```python
from build123d import *

# Parameters (mm, degrees)
SKETCH1_R           = 12.7
BOSS_EXTRUDE1_DEPTH = 12.7
SKETCH2_R           = 1.6256
CUT_EXTRUDE1_DEPTH  = 9.525
SKETCH3_R           = 9.525
CUT_EXTRUDE2_DEPTH  = 2.54
BOSS_EXTRUDE6_START = -12.7
BOSS_EXTRUDE6_DEPTH = 12.7
SKETCH15_R          = 12.7
BOSS_EXTRUDE8_DEPTH = 12.7
SKETCH17_R          = 1.651
CUT_EXTRUDE4_DEPTH  = 12.7
SKETCH18_R          = 3.81
CUT_EXTRUDE5_DEPTH  = 10.9027722
SKETCH19_R          = 8.255
CUT_EXTRUDE6_DEPTH  = 8.3627722
SKETCH20_R          = 9.525
CUT_EXTRUDE7_DEPTH  = 5.1877722
SKETCH21_R          = 1.2192
CUT_EXTRUDE8_DEPTH  = 4.3372278


with BuildPart() as part:
    # Sketch1 → Boss-Extrude1 (new body)
    with BuildSketch(Plane(origin=(0, 0, 0), x_dir=(1, 0, 0), z_dir=(0, 1, 0))):
        with Locations(Location((0, 0, 0), (0, 0, 270))):
            Circle(SKETCH1_R)
    extrude(amount=BOSS_EXTRUDE1_DEPTH)

    # Sketch2 → Cut-Extrude1 (cut)
    with BuildSketch(Plane.XZ):
        with Locations(Location((0, 0, 0), (0, 0, 270))):
            Circle(SKETCH2_R)
    extrude(amount=-CUT_EXTRUDE1_DEPTH, mode=Mode.SUBTRACT)

    # Sketch3 → Cut-Extrude2 (cut)
    with BuildSketch(Plane.XZ):
        with Locations(Location((0, 0, 0), (0, 0, 270))):
            Circle(SKETCH3_R)
    extrude(amount=-CUT_EXTRUDE2_DEPTH, mode=Mode.SUBTRACT)

    # Sketch14 → Boss-Extrude6 (add)
    with BuildSketch(Plane(origin=(0, 12.7, 0), x_dir=(1, 0, 0), z_dir=(0, 1, 0)).offset(BOSS_EXTRUDE6_START)):
        with BuildLine():
            Line((15.875, 12.7), (0, 12.7))
            ThreePointArc((0, 12.7), (8.980256121, 8.980256121), (12.7, 0))
            ThreePointArc((12.7, 0), (8.980256121, -8.980256121), (0, -12.7))
            Line((0, -12.7), (15.875, -12.7))
            Line((15.875, -12.7), (15.875, 12.7))
        make_face()
    extrude(amount=BOSS_EXTRUDE6_DEPTH)

    # Sketch5 → #2-56 Tapped Hole1 (revolve, cut)
    with BuildSketch(Plane(origin=(0, 3.81, 0), x_dir=(0, 1, 0), z_dir=(1, 0, 0))):
        Polygon((0, 0), (0, 13.74216509), (0.889, 13.208), (0.889, 0), align=None)
    revolve(axis=Axis((0, 3.81, -6.35), (0, 0, 1)), mode=Mode.SUBTRACT)

    # Sketch15 → Boss-Extrude8 (add)
    with BuildSketch(Plane(origin=(15.875, 0, 0), x_dir=(0, 0, -1), z_dir=(1, 0, 0))):
        with Locations((0, 25.4)):
            Circle(SKETCH15_R)
        with BuildLine():
            ThreePointArc((0, 12.7), (-8.980256121, 16.419743879), (-12.7, 25.4))
            Line((-12.7, 25.4), (-12.7, 12.7))
            Line((-12.7, 12.7), (0, 12.7))
        make_face()
        with BuildLine():
            Line((12.7, 12.7), (12.7, 25.4))
            ThreePointArc((12.7, 25.4), (8.980256121, 16.419743879), (0, 12.7))
            Line((0, 12.7), (12.7, 12.7))
        make_face()
    extrude(amount=-BOSS_EXTRUDE8_DEPTH)

    # Sketch17 → Cut-Extrude4 (cut)
    with BuildSketch(Plane.ZY.offset(-3.175)):
        with Locations((0, 25.4)):
            Circle(SKETCH17_R)
    extrude(amount=-CUT_EXTRUDE4_DEPTH, mode=Mode.SUBTRACT)

    # Sketch18 → Cut-Extrude5 (cut)
    with BuildSketch(Plane.ZY.offset(-3.175)):
        with Locations((0, 25.4)):
            Circle(SKETCH18_R)
    extrude(amount=-CUT_EXTRUDE5_DEPTH, mode=Mode.SUBTRACT)

    # Sketch19 → Cut-Extrude6 (cut)
    with BuildSketch(Plane.ZY.offset(-3.175)):
        with Locations((0, 25.4)):
            Circle(SKETCH19_R)
    extrude(amount=-CUT_EXTRUDE6_DEPTH, mode=Mode.SUBTRACT)

    # Sketch20 → Cut-Extrude7 (cut)
    with BuildSketch(Plane.ZY.offset(-3.175)):
        with Locations((0, 25.4)):
            Circle(SKETCH20_R)
    extrude(amount=-CUT_EXTRUDE7_DEPTH, mode=Mode.SUBTRACT)

    # Sketch21 → Cut-Extrude8 (cut)
    with BuildSketch(Plane.ZY.offset(-11.5377722)):
        with Locations((5.4599967, 25.4)):
            Circle(SKETCH21_R)
        with Locations((-5.4599967, 25.4)):
            Circle(SKETCH21_R)
    extrude(amount=-CUT_EXTRUDE8_DEPTH, mode=Mode.SUBTRACT)


solid = part.part
```
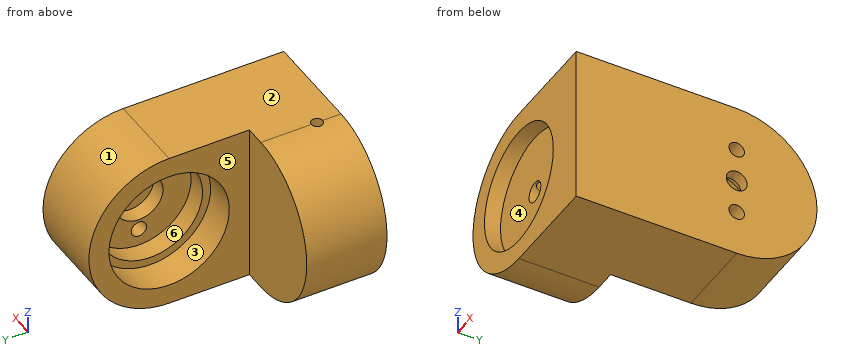
Design review of the part built by this model. Coordinates are the model's own, in mm. Face numbers are marked on the shaded views. A direction names the side the tool comes from. Round coordinates to 2 decimals unless told otherwise and drop trailing zeros. Write each loop counter-clockwise with the first axis right and the second up, starting at its lowest first coordinate (ties: lowest second). Pieces come first, ordered by that corner, then holes. Notation, with made-up numbers: (0, 77) -> (4, 77) arc R13 ccw to (4, 85) -> close; hole circle Ø6 at (75.5, 11.25). An arc over 180 degrees is marked (long way). Answer in a Markdown table with one row per item.
Q1. Draft analysis for pull direction Y (two halves, no side actions). For the marked faces 1, 2 and 3, state which applies: +Y half, -Y half, draft (parallel to the pull), parting line (faces both ways), or undercut.
The answers:
| item | result |
|---|---|
| face 1 | +Y half |
| face 2 | draft |
| face 3 | undercut |
Q2. For the marked faces 4, 5 and 6, list the 3-axis set-ups (+Z, -Z, +X, -X, +Y, -Y) from which the entire face can be reached by the end or side of a thin tool; tool diameter is ignored.
The answers:
| item | result |
|---|---|
| face 4 | -Y |
| face 5 | +Z, -Z, -X, +Y |
| face 6 | -X |
Q3. To check wall thickness, follow L1, parallel to Y at x = 15.3, z = 0; L2, parallel to Y at x = 12.3, z = 0; L3, parallel to X at y = 21, z = 2.75 (3 decimals). State the ranges of each line that lie inside material, in increasing order. Write a range as [from, to].
The answers:
| item | result |
|---|---|
| L1 | [0, 23.75], [27.05, 38.1] |
| L2 | [0, 21.59], [29.21, 38.1] |
| L3 | [11.538, 15.875] |
Q4. Take a section at B-B, the plane x = 12.75. State the section outline as (y, z) points.
The answers:
| item | result |
|---|---|
| outline | (0, -12.7) -> (25.4, -12.7) arc R12.7 ccw to (25.4, 12.7) -> (0, 12.7) -> close; hole circle Ø7.62 at (25.4, 0); hole circle Ø2.44 at (25.4, -5.46); hole circle Ø2.44 at (25.4, 5.46) |
Q5. Clearance check with flat-ended pins moving along their axes: pin 1 Ø12.5 at (y, z) = (22.5, 4) entering from -X (3 decimals); pin 2 Ø6 at (y, z) = (25.4, 0) entering from -X; pin 3 Ø4 at (x, z) = (0, 0) entering from +Y. State where each tip first meets the part, or that it passes through.
The answers:
| item | result |
|---|---|
| pin 1 | x = 3.175 |
| pin 2 | x = 14.08 |
| pin 3 | y = 12.7 |
Q6. Take a section at D-D, the plane y = 23. State the section outline as (x, z) points (3 decimals), then the cut area to 3 significant figures.
The answers:
| item | result |
|---|---|
| outline | (3.175, -12.7) -> (15.875, -12.7) -> (15.875, 12.7) -> (3.175, 12.7) -> (3.175, 9.218) -> (8.363, 9.218) -> (8.363, 7.898) -> (11.538, 7.898) -> (11.538, 2.959) -> (14.078, 2.959) -> (14.078, -2.959) -> (11.538, -2.959) -> (11.538, -7.898) -> (8.363, -7.898) -> (8.363, -9.218) -> (3.175, -9.218) -> close |
| area | 162 mm² |
Q7. Take a section at C-C, the plane x = 7. State the section outline as (y, z) points (3 decimals).
The answers:
| item | result |
|---|---|
| outline | (0, -12.7) -> (25.4, -12.7) arc R12.7 ccw to (25.4, 12.7) -> (0, 12.7) -> (0, 6.46) -> (2.54, 6.46) -> (2.54, -6.46) -> (0, -6.46) -> close; hole circle Ø19.05 at (25.4, 0) |
